Check sheet for the modelled part. Datum: model origin and axes. Units: mm. Give positions to 0.01 mm unless a question says otherwise; leave off trailing zeros. Order: outer loops, then holes, each group sorted by start corner. A loop starts at its lowest first (then second) coordinate and runs counter-clockwise, first axis right, second up. Notation, with made-up numbers: M -25.5,-26.75 L 12.5,-26.75 A30 cw 12.5,11.25 Z; hole C 51,5 d6. An arc over 180 degrees is marked long. Answer in a Markdown table with one row per item. Add a question column.
Autodesk Inventor part; units mm, degrees
ref_plane "YZ Plane" through (0, 0, 0) normal (1, 0, 0) x (0, 1, 0)
ref_plane "XZ Plane" through (0, 0, 0) normal (0, 1, 0) x (-1, 0, 0)
ref_plane "XY Plane" through (0, 0, 0) normal (0, 0, 1) x (1, 0, 0)
sketch "Sketch1" plane through (0, 0, 0) normal (0, 1, 0) x (-1, 0, 0)
  line L0 (-38, -107) -> (38, -107)
  line L1 (38, -107) -> (38, 107)
  line L2 (38, 107) -> (-38, 107)
  line L3 (-38, 107) -> (-38, -107)
  line L4 (-38, -107) -> (38, 107) construction
  line L5 (38, -107) -> (-38, 107) construction
  point P0 (0, 0)
  dimension "d0" = 76
  dimension "d1" = 214
extrude "Extrusion1" add sketch "Sketch1" against normal blind 3
sketch "Sketch2" plane through (0, -3, 0) normal (0, -1, 0) x (1, 0, 0)
  line L0 (-38, 107) -> (-38, -107)
  line L1 (-38, -107) -> (38, -107)
  line L2 (38, -107) -> (38, 107)
  line L3 (38, 107) -> (-38, 107)
  line L4 (35, 104) -> (-35, 104)
  line L5 (-35, 104) -> (-35, -104)
  line L6 (-35, -104) -> (35, -104)
  line L7 (35, -104) -> (35, 104)
  line L8 (35, 104) -> (-35, -104) construction
  line L9 (-35, 104) -> (35, -104) construction
  point P0 (0, 0)
  dimension "d4" = 3
  dimension "d5" = 3
extrude "Extrusion2" add sketch "Sketch2" along normal blind 3 contours L7 L6 L5 L4
fillet "Fillet1" radius 2 8 edges at (35, -4.5, 104) (-35, -4.5, 104) (38, -1.5, 107) (-38, -1.5, 107) (35, -4.5, -104) (38, -1.5, -107) (-35, -4.5, -104) (-38, -1.5, -107)
properties part number "module-lid_command"
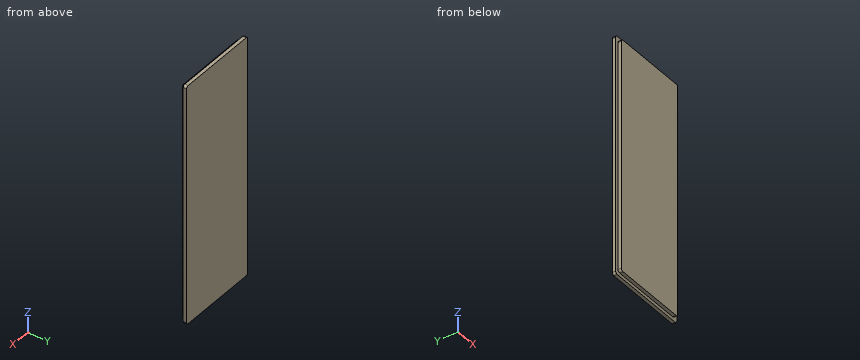
Q1. Cross-section at B-B (z = -40). Record the boundary of the cut face in (x, y), and give its area (3 significant figures).
Q2. Go/stop test with flat-tipped pins: pin 1 (2.5 mm diameter, centred on y = -4, z = 30.5, fed in from +X); pin 2 (0.9 mm diameter, centred on y = -4, z = 7, fed in from -X); pin 3 (0.9 mm diameter, centred on x = -2.5, y = -4.5, fed in from -Z); pin 4 (1.5 mm diameter, centred on x = -12.5, y = -5, fed in from +Z). Record where each tip stops, or that it passes through.
Q3. Thickness scan on probe 1 along Z at (x, y) = (-18.5, -5.15); probe 2 along X at (y, z) = (-5.2, 92). Record the ranges inside material, lowest first.
Q4. Cross-section at A-A (y = -4.75). Record the boundary of the cut face in (x, z), and give its area (3 significant figures).
Values follow:
| question | item | result |
|---|---|---|
| 1 | outline | M -38,-3 L -35,-3 L -35,-6 L 35,-6 L 35,-3 L 38,-3 L 38,0 L -38,0 Z |
| 1 | area | 438 mm² |
| 2 | pin 1 | x = 38 |
| 2 | pin 2 | x = -35 |
| 2 | pin 3 | z = -104 |
| 2 | pin 4 | z = 104 |
| 3 | probe 1 | -104 to 104 |
| 3 | probe 2 | -35 to 35 |
| 4 | outline | M -35,-102 A2 ccw -33,-104 L 33,-104 A2 ccw 35,-102 L 35,102 A2 ccw 33,104 L -33,104 A2 ccw -35,102 Z |
| 4 | area | 14,600 mm² |
